Verification items for the finished model (mm, model axes). Face numbers are marked on the shaded views. A direction names the side the tool comes from. Round coordinates to 2 decimals unless told otherwise and drop trailing zeros. Order: outer loops, then holes, each group sorted by start corner. A loop starts at its lowest first (then second) coordinate and runs counter-clockwise, first axis right, second up. Notation, with made-up numbers: (-37, -25.5) -> (-29, -25.5) arc R26 cw to (-29, 8.5) -> close; hole circle Ø1 at (12.5, -15). An arc over 180 degrees is marked (long way). Write item = value, one per line. Start each with the question number.
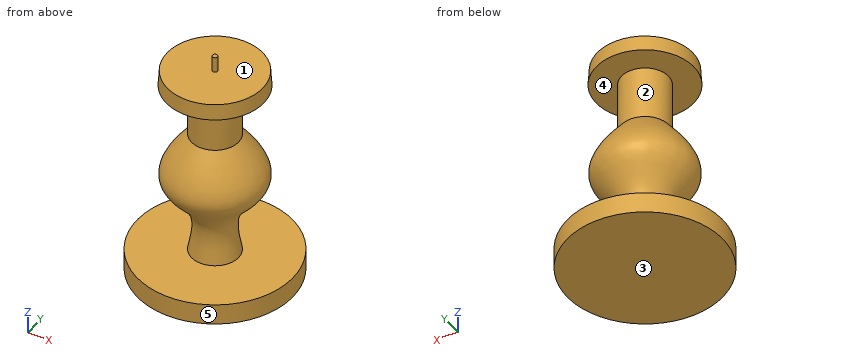
from build123d import *

# Parameters (mm, degrees)
F0_W   = 13.291821114
F0_H   = 5.08
F0_W_2 = 0.6099150633
F0_H_2 = 3.8282163441


with BuildPart() as f1:
    # F0 (on Front) → F1 (revolve)
    with BuildSketch(Plane.XZ):
        with Locations((-12.404089443, -72.1843269592)):
            Rectangle(F0_W, F0_H)
        Polygon((-5.758178886, -69.6443269592), (-5.758178886, -74.7243269592), (-4.7780917957, -74.7243269592), (0, -74.7243269592), (0, -69.6443269592), align=None)
        with BuildLine():
            add(Edge.make_bspline(
                [(-5.758178886, -69.6443269592), (-4.9648323817, -65.7790976541), (-3.4035942307, -58.1726565582), (-15.3237312615, -50.8868167952), (-9.0760322015, -43.097913485), (-5.758178886, -38.9616005123)],
                knots=[0, 0, 0, 0, 0.3263693982, 0.6422670964, 1, 1, 1, 1], degree=3))
            Line((-5.758178886, -69.6443269592), (0, -69.6443269592))
            Line((0, -69.6443269592), (0, -22.2111493349))
            Line((0, -22.2111493349), (-0.6099150633, -22.2111493349))
            Line((-0.6099150633, -22.2111493349), (-11.6852605715, -22.2111493349))
            Line((-11.6852605715, -22.2111493349), (-11.9429603219, -26.0766372085))
            Line((-11.9429603219, -26.0766372085), (-5.758178886, -26.0766372085))
            Line((-5.758178886, -26.0766372085), (-5.758178886, -38.9616005123))
        make_face()
        with Locations((-0.3049575316, -20.2970411628)):
            Rectangle(F0_W_2, F0_H_2)
    revolve(axis=Axis((0, 0, -0.6833137407), (0, 0, -1)))


solid = f1.part
(1) Draft check along Z on the marked faces 1, 2 and 3. Enter one of: +Z half, -Z half, draft (parallel to the pull), parting line (faces both ways), or undercut.
(2) Set-up check for the marked faces 4 and 5: record each of +Z, -Z, +X, -X, +Y, -Y from which the full face is reachable in a straight line by a thin tool's end or side.
(3) Cross-section at A-A (y = 9.5). Give the number of separate pieces and of enclosed holes in the cut face, and give its area (3 significant figures).
(4) Scan lines: line 1 along Z through (x, y) = (10, -2.5); line 2 along Z through (x, y) = (6, 3.5); line 3 along Z through (x, y) = (16, -6). Record each from-to range of solid material in increasing order. Write a range as from..to.
(5) Cross-section at B-B (z = -70.5). Enter the section's corners in (x, y).
(6) Cross-section at C-C (x = -14). Enter the section's corners in (y, z).
(7) Cross-section at D-D (y = -15.5). Enter the section's corners in (x, z), and give its area (3 significant figures).
(8) Depth check by flat-ended pin: pin 1 (8 mm diameter, centred on x = 14, y = 5, fed in from +Z); pin 2 (4 mm diameter, centred on x = 6.5, y = -13, fed in from +Z); pin 3 (6 mm diameter, centred on x = -11, z = -30, fed in from -Y). Enter the tip coordinate at first touch or a pass-through.
Outcome:
q1.face_1 = +Z half
q1.face_2 = undercut
q1.face_3 = -Z half
q2.face_4 = none
q2.face_5 = +Z, -Z
q3.separate_pieces = 3
q3.enclosed_holes = 0
q3.area = 331 mm^2
q4.line_1 = -74.72..-69.64, -53.21..-45.2, -26.08..-22.21
q4.line_2 = -74.72..-69.64, -57.02..-40.45, -26.08..-22.21
q4.line_3 = -74.72..-69.64
q5.outline = circle Ø38.1 at (0, 0)
q6.outline = (-12.92, -74.72) -> (12.92, -74.72) -> (12.92, -69.64) -> (-12.92, -69.64) -> close
q7.outline = (-11.07, -74.72) -> (11.07, -74.72) -> (11.07, -69.64) -> (-11.07, -69.64) -> close
q7.area = 113 mm^2
q8.pin_1 = -22.21
q8.pin_2 = -69.64
q8.pin_3 = through
